```python
from build123d import *

# Parameters (mm, degrees)
SKETCH1_R           = 152.4
BOSS_EXTRUDE1_DEPTH = 101.6
CUT_EXTRUDE1_DEPTH  = 102.6
BOSS_EXTRUDE3_DEPTH = 101.6


with BuildPart() as part:
    # Sketch1 → Boss-Extrude1 (new body)
    with BuildSketch(Plane.XY):
        Circle(SKETCH1_R)
    extrude(amount=BOSS_EXTRUDE1_DEPTH)

    # Sketch2 → Cut-Extrude1 (cut, through all)
    with BuildSketch(Plane.XY.offset(101.6)):
        with BuildLine():
            Line((-7.62, 50.225248631), (-7.62, 58.42))
            Line((-7.62, 58.42), (7.62, 58.42))
            Line((7.62, 58.42), (7.62, 50.225248631))
            ThreePointArc((7.62, 50.225248631), (0, -50.8), (-7.62, 50.225248631))
        make_face()
    extrude(amount=-CUT_EXTRUDE1_DEPTH, mode=Mode.SUBTRACT)

    # Sketch3 → Boss-Extrude3 (add)
    with BuildSketch(Plane.XY.offset(101.6)):
        with BuildLine():
            Line((0.984560076, 177.011085759), (11.138596509, 176.66302813))
            ThreePointArc((11.138596509, 176.66302813), (15.196562883, 164.436371227), (15.869603853, 151.571487007))
            ThreePointArc((15.869603853, 151.571487007), (5.22086444, 152.310546498), (-5.453487698, 152.302394833))
            ThreePointArc((-5.453487698, 152.302394833), (-3.901102684, 165.090996434), (0.984560076, 177.011085759))
        make_face()
        with BuildLine():
            Line((44.974495255, 171.205106866), (54.722965549, 168.342777932))
            ThreePointArc((54.722965549, 168.342777932), (55.612797522, 155.491068739), (53.065327067, 142.862980031))
            ThreePointArc((53.065327067, 142.862980031), (42.934934006, 146.227054412), (32.593909032, 148.873762275))
            ThreePointArc((32.593909032, 148.873762275), (37.277918906, 160.874523986), (44.974495255, 171.205106866))
        make_face()
        with BuildLine():
            Line((86.138517492, 154.641681459), (94.868889406, 149.444931875))
            ThreePointArc((94.868889406, 149.444931875), (92.534675563, 136.775690545), (86.926760621, 125.177866606))
            ThreePointArc((86.926760621, 125.177866606), (77.951243764, 130.955578711), (68.593310586, 136.090843714))
            ThreePointArc((68.593310586, 136.090843714), (76.114631752, 146.549713541), (86.138517492, 154.641681459))
        make_face()
        with BuildLine():
            Line((121.890139881, 128.361550474), (129.053852039, 121.156911128))
            ThreePointArc((129.053852039, 121.156911128), (123.642259619, 109.46619269), (115.326266111, 99.62736745))
            ThreePointArc((115.326266111, 99.62736745), (108.069590193, 107.455682379), (100.282742167, 114.756836935))
            ThreePointArc((100.282742167, 114.756836935), (110.168782355, 123.016645622), (121.890139881, 128.361550474))
        make_face()
        with BuildLine():
            Line((149.9829565, 94.015991192), (155.129886522, 85.256156071))
            ThreePointArc((155.129886522, 85.256156071), (146.980945779, 75.278531359), (136.47939816, 67.816914393))
            ThreePointArc((136.47939816, 67.816914393), (131.397526817, 77.203950329), (125.671040244, 86.212236046))
            ThreePointArc((125.671040244, 86.212236046), (137.30062319, 91.753989435), (149.9829565, 94.015991192))
        make_face()
        with BuildLine():
            Line((168.651792363, 53.763061417), (171.458539706, 43.998443178))
            ThreePointArc((171.458539706, 43.998443178), (161.084278558, 36.360843047), (149.057027687, 31.745275192))
            ThreePointArc((149.057027687, 31.745275192), (146.469273585, 42.101210144), (143.162964676, 52.250603299))
            ThreePointArc((143.162964676, 52.250603299), (155.805360914, 54.726092645), (168.651792363, 53.763061417))
        make_face()
        with BuildLine():
            Line((176.723615855, 10.132000766), (177.01382226, -0.023853715))
            ThreePointArc((177.01382226, -0.023853715), (165.066093688, -4.841530759), (152.268855971, -6.3210364))
            ThreePointArc((152.268855971, -6.3210364), (152.337817217, 4.353096088), (151.659433521, 15.005872983))
            ThreePointArc((151.659433521, 15.005872983), (164.520274799, 14.259554184), (176.723615855, 10.132000766))
        make_face()
        with BuildLine():
            Line((173.691244618, -34.135690756), (171.446675351, -44.044651791))
            ThreePointArc((171.446675351, -44.044651791), (158.676199082, -45.739693381), (145.913072029, -43.990174028))
            ThreePointArc((145.913072029, -43.990174028), (148.634415534, -33.668539005), (150.626582394, -23.181731521))
            ThreePointArc((150.626582394, -23.181731521), (162.897774756, -27.102964508), (173.691244618, -34.135690756))
        make_face()
        with BuildLine():
            Line((159.74521369, -76.258511285), (155.106903292, -85.297962411))
            ThreePointArc((155.106903292, -85.297962411), (142.316095317, -83.76386285), (130.389033141, -78.895247238))
            ThreePointArc((130.389033141, -78.895247238), (135.591766884, -69.574655969), (140.129309129, -59.912742576))
            ThreePointArc((140.129309129, -59.912742576), (151.039808429, -66.762504263), (159.74521369, -76.258511285))
        make_face()
        with BuildLine():
            Line((135.761803484, -113.589729091), (129.021194056, -121.191688348))
            ThreePointArc((129.021194056, -121.191688348), (117.013747881, -116.524840753), (106.672171762, -108.843041907))
            ThreePointArc((106.672171762, -108.843041907), (114.02938885, -101.109141419), (120.827196012, -92.879215672))
            ThreePointArc((120.827196012, -92.879215672), (129.691455452, -102.227110339), (135.761803484, -113.589729091))
        make_face()
        with BuildLine():
            Line((103.247979869, -143.783686465), (94.828608691, -149.470494794))
            ThreePointArc((94.828608691, -149.470494794), (84.358996319, -141.964134364), (76.25270552, -131.951827956))
            ThreePointArc((76.25270552, -131.951827956), (85.302124943, -126.290567662), (93.933065798, -120.009746062))
            ThreePointArc((93.933065798, -120.009746062), (100.194111358, -131.268411108), (103.247979869, -143.783686465))
        make_face()
        with BuildLine():
            Line((64.246705958, -164.943186018), (54.677593087, -168.357520338))
            ThreePointArc((54.677593087, -168.357520338), (46.403658768, -158.483299305), (41.042001351, -146.76959537))
            ThreePointArc((41.042001351, -146.76959537), (51.215014806, -143.536693073), (61.136775598, -139.599622741))
            ThreePointArc((61.136775598, -139.599622741), (64.401202759, -152.061634836), (64.246705958, -164.943186018))
        make_face()
        with BuildLine():
            Line((21.20857523, -175.738698575), (11.090983218, -176.666023704))
            ThreePointArc((11.090983218, -176.666023704), (5.532608676, -165.04437569), (3.252477296, -152.365289326))
            ThreePointArc((3.252477296, -152.365289326), (13.909876934, -151.763880168), (24.499036942, -150.417941712))
            ThreePointArc((24.499036942, -150.417941712), (24.561729739, -163.300266803), (21.20857523, -175.738698575))
        make_face()
        with BuildLine():
            Line((-23.16216828, -175.49190238), (-33.192513915, -173.873951069))
            ThreePointArc((-33.192513915, -173.873951069), (-35.686075567, -161.23510696), (-34.74141187, -148.387311794))
            ThreePointArc((-34.74141187, -148.387311794), (-24.269269663, -150.455184524), (-13.678066306, -151.784948207))
            ThreePointArc((-13.678066306, -151.784948207), (-16.821047091, -164.27814243), (-23.16216828, -175.49190238))
        make_face()
        with BuildLine():
            Line((-66.077547573, -164.218304543), (-75.390403326, -160.156738624))
            ThreePointArc((-75.390403326, -160.156738624), (-74.662472438, -147.294843478), (-70.552370357, -135.085613731))
            ThreePointArc((-70.552370357, -135.085613731), (-60.923488791, -139.6928363), (-50.995726343, -143.61474818))
            ThreePointArc((-50.995726343, -143.61474818), (-57.14689567, -154.933818196), (-66.077547573, -164.218304543))
        make_face()
        with BuildLine():
            Line((-104.841031535, -142.62626668), (-112.851236429, -136.376289276))
            ThreePointArc((-112.851236429, -136.376289276), (-108.947551576, -124.099503267), (-101.930263942, -113.295989747))
            ThreePointArc((-101.930263942, -113.295989747), (-93.749661058, -120.153073417), (-85.109137346, -126.420705346))
            ThreePointArc((-85.109137346, -126.420705346), (-93.881994622, -135.854432358), (-104.841031535, -142.62626668))
        make_face()
        with BuildLine():
            Line((-137.016967907, -112.072495938), (-143.22121131, -104.026816116))
            ThreePointArc((-143.22121131, -104.026816116), (-136.387055368, -93.106534861), (-126.90350417, -84.387562054))
            ThreePointArc((-126.90350417, -84.387562054), (-120.685197332, -93.06365104), (-113.874828239, -101.283184653))
            ThreePointArc((-113.874828239, -101.283184653), (-124.718142578, -108.238812898), (-137.016967907, -112.072495938))
        make_face()
        with BuildLine():
            Line((-160.583624273, -74.476798103), (-164.592070753, -65.140955515))
            ThreePointArc((-164.592070753, -65.140955515), (-155.256858874, -56.263340447), (-143.902930513, -50.176753481))
            ThreePointArc((-143.902930513, -50.176753481), (-140.03763881, -60.126697203), (-135.485344872, -69.781668975))
            ThreePointArc((-135.485344872, -69.781668975), (-147.717790955, -73.822150748), (-160.583624273, -74.476798103))
        make_face()
        with BuildLine():
            Line((-174.06022094, -32.201449136), (-175.621005064, -22.162049108))
            ThreePointArc((-175.621005064, -22.162049108), (-164.371302942, -15.884913431), (-151.860406493, -12.81315495))
            ThreePointArc((-151.860406493, -12.81315495), (-150.591000419, -23.411761851), (-148.582819006, -33.895514396))
            ThreePointArc((-148.582819006, -33.895514396), (-161.435787258, -34.766971368), (-174.06022094, -32.201449136))
        make_face()
        with BuildLine():
            Line((-176.599973777, 12.097235308), (-175.615025737, 22.209380351))
            ThreePointArc((-175.615025737, 22.209380351), (-163.157693531, 25.491621116), (-150.27593463, 25.35554123))
            ThreePointArc((-150.27593463, 25.35554123), (-151.682175636, 14.774220601), (-152.344288173, 4.120420012))
            ThreePointArc((-152.344288173, 4.120420012), (-165.010179328, 6.472744687), (-176.599973777, 12.097235308))
        make_face()
        with BuildLine():
            Line((-168.043300773, 55.635805968), (-164.574508477, 65.185312762))
            ThreePointArc((-164.574508477, 65.185312762), (-151.692286184, 65.266423358), (-139.249073118, 61.931055503))
            ThreePointArc((-139.249073118, 61.931055503), (-143.24260191, 52.031884437), (-146.533405431, 41.877453276))
            ThreePointArc((-146.533405431, 41.877453276), (-158.216374966, 47.305754388), (-168.043300773, 55.635805968))
        make_face()
        with BuildLine():
            Line((-148.92784916, 95.678574324), (-143.193169586, 104.065412237))
            ThreePointArc((-143.193169586, 104.065412237), (-130.695494611, 100.940296186), (-119.47268022, 94.615213793))
            ThreePointArc((-119.47268022, 94.615213793), (-125.802568697, 86.020193614), (-131.515289913, 77.003172136))
            ThreePointArc((-131.515289913, 77.003172136), (-141.481253886, 85.166369563), (-148.92784916, 95.678574324))
        make_face()
        with BuildLine():
            Line((-120.454713067, 129.709505975), (-112.814477223, 136.406699136))
            ThreePointArc((-112.814477223, 136.406699136), (-101.486624446, 130.271718973), (-92.189379433, 121.35435023))
            ThreePointArc((-92.189379433, 121.35435023), (-100.457897423, 114.603537665), (-108.233585051, 107.290498494))
            ThreePointArc((-108.233585051, 107.290498494), (-115.856345292, 117.675668518), (-120.454713067, 129.709505975))
        make_face()
        with BuildLine():
            Line((-84.41296435, 155.590312327), (-75.347236353, 160.17705146))
            ThreePointArc((-75.347236353, 160.17705146), (-65.900976426, 151.417690551), (-59.113480889, 140.468346531))
            ThreePointArc((-59.113480889, 140.468346531), (-68.801086995, 135.985919963), (-78.151165985, 130.836368244))
            ThreePointArc((-78.151165985, 130.836368244), (-82.951756434, 142.790972439), (-84.41296435, 155.590312327))
        make_face()
        with BuildLine():
            Line((-43.067238634, 171.694807134), (-33.145651515, 173.88289055))
            ThreePointArc((-33.145651515, 173.88289055), (-26.174527691, 163.049531756), (-22.323264935, 150.756200014))
            ThreePointArc((-22.323264935, 150.756200014), (-32.821251239, 148.823806789), (-43.15822174, 146.161307795))
            ThreePointArc((-43.15822174, 146.161307795), (-44.835003644, 158.934194413), (-43.067238634, 171.694807134))
        make_face()
    extrude(amount=-BOSS_EXTRUDE3_DEPTH)


solid = part.part
```
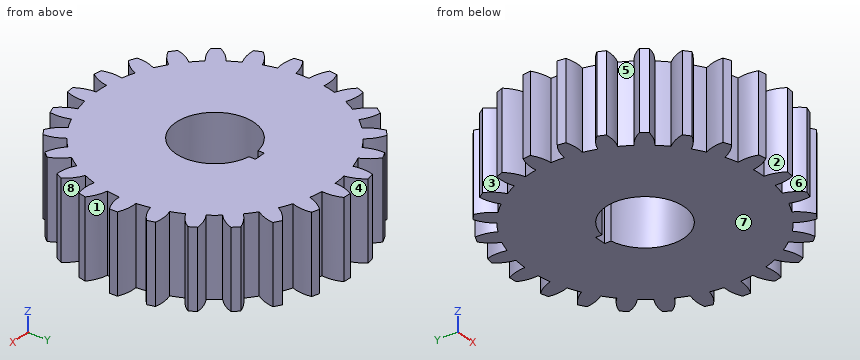
For this review, take the finished solid that the model builds, in its own axes (mm). Face numbers are marked on the shaded views. A direction names the side the tool comes from. Coordinates: 2 decimals unless noted, no trailing zeros. Answer in a Markdown table with one row per item. Add a question column.
Q1. Draft analysis for pull direction Y (two halves, no side actions). For the marked faces 6, 7 and 8, state which applies: +Y half, -Y half, draft (parallel to the pull), parting line (faces both ways), or undercut.
Q2. Tool access review of the marked faces 1, 2, 3, 4 and 5: name each direction out of +Z, -Z, +X, -X, +Y, -Y from which nothing blocks a thin tool from reaching the whole face with its end or side.
Q3. For probe 1 along X at (y, z) = (0, 71); probe 2 along X at (y, z) = (46.5, 67); probe 3 along Y at (x, z) = (0, 74), list the stretches that pass through material, from the lowest coordinate up.
Q4. For P1, Ø6.5, axis at y = 55, z = 29.5, coming from the -X side; P2, Ø12, axis at y = -4.5, z = 88, coming from the -X side; P3, Ø6.5, axis at y = 54.5, z = 43.5, coming from the +X side, all flat-tipped, find the tip position at first contact; note any pin that passes through.
Answer list:
| question | item | result |
|---|---|---|
| 1 | face 6 | -Y half |
| 1 | face 7 | draft |
| 1 | face 8 | undercut |
| 2 | face 1 | +Z, -Z, +X |
| 2 | face 2 | +Z, -Z, -Y |
| 2 | face 3 | +Z, -Z, -X |
| 2 | face 4 | +Z, -Z, +Y |
| 2 | face 5 | +Z, -Z |
| 3 | probe 1 | x = -152.4 to -50.8, 50.8 to 177.01 |
| 3 | probe 2 | x = -156.91 to -20.45, 20.45 to 170.74 |
| 3 | probe 3 | y = -152.4 to -50.8, 58.42 to 175.22 |
| 4 | P1 | stops at x = -168.04 |
| 4 | P2 | stops at x = -152.4 |
| 4 | P3 | stops at x = 169.37 |
